Autodesk Inventor part; units mm, degrees
ref_plane "YZ Plane" through (0, 0, 0) normal (1, 0, 0) x (0, 1, 0)
ref_plane "XZ Plane" through (0, 0, 0) normal (0, 1, 0) x (-1, 0, 0)
ref_plane "XY Plane" through (0, 0, 0) normal (0, 0, 1) x (1, 0, 0)
sketch "Sketch1" plane through (0, 0, 0) normal (0, 0, 1) x (1, 0, 0)
  line L0 (-40.9154, -1.8235) -> (49.0846, -1.8235)
  line L1 (49.0846, -1.8235) -> (49.0846, -3.8235)
  line L2 (49.0846, -3.8235) -> (-40.9154, -3.8235)
  line L3 (-40.9154, -3.8235) -> (-40.9154, -1.8235)
  line L4 (-40.9154, -1.8235) -> (-33.9154, -1.8235)
  line L5 (-33.9154, -1.8235) -> (-33.9154, 15.1765)
  line L6 (-33.9154, 15.1765) -> (-40.9154, 15.1765)
  line L7 (-40.9154, 15.1765) -> (-40.9154, -1.8235)
  line L8 (49.0846, -1.8235) -> (43.0846, -1.8235)
  line L9 (43.0846, -1.8235) -> (43.0846, 15.1765)
  line L10 (43.0846, 15.1765) -> (49.0846, 15.1765)
  line L11 (49.0846, 15.1765) -> (49.0846, -1.8235)
  circle A0 centre (-36.9154, 6.1765) radius 1.5
  circle A1 centre (46.0846, 11.1765) radius 1.5
  circle A2 centre (46.0846, 1.1765) radius 1.5
  point P0 (0, 0)
  point P1 (43.0846, -1.8235)
  point P2 (43.0846, -1.8235)
  dimension "d0" = 2
  dimension "d1" = 90
  dimension "d2" = 10
  dimension "d3" = 5
  dimension "d4" = 15
  dimension "d5" = 83
  dimension "d6" = 83
  dimension "d7" = 4
  dimension "d8" = 3
  dimension "d9" = 3
  dimension "d10" = 3
  dimension "d11" = 19
  dimension "d12" = 3
  dimension "d13" = 3
  dimension "d14" = 3
extrude "Extrusion1" add sketch "Sketch1" against normal blind 10 contours L7 L6 L5 L0 | L0 L1 L2 L3 | L9 L10 L11 L0 | A0 | A1 | A2
fillet "Fillet1" radius 2 2 edges at (-37.4154, 15.1765, 0) (46.0846, 15.1765, 0)
sketch "Sketch2" plane through (0, 0, 0) normal (0, 0, 1) x (1, 0, 0)
  line L0 (-40.9154, -3.8235) -> (49.0846, -3.8235)
  line L1 (-40.9154, 13.1765) -> (-40.9154, -3.8235)
  line L2 (49.0846, -3.8235) -> (49.0846, 13.1765)
  point P0 (0, 0)
  point P1 (-36.9154, 6.1765)
  point P2 (46.0846, 1.1765)
  point P3 (46.0846, 11.1765)
  dimension "d18" = 10
  dimension "d19" = 5
  dimension "d20" = 15
  dimension "d21" = 4
  dimension "d22" = 83
  dimension "d23" = 83
  dimension "d24" = 3
hole "Hole1" at (-36.9154, 6.1765, 0) at (46.0846, 1.1765, 0) at (46.0846, 11.1765, 0) direction (0, 0, -1) diameter 3 depth 10 tip angle 118
chamfer "Chamfer1" distance 2 angle 45 2 edges at (-33.9154, -1.8235, -5) (43.0846, -1.8235, -5)
sketch "Sketch3" plane through (-31.9154, -1.8235, 0) normal (0, 1, 0) x (1, 0, 0)
  line L0 (73, 0) -> (0, 0)
  line L1 (73, 10) -> (73, 0)
  point P0 (31.9154, 0)
  point P1 (23, 3.2)
  point P2 (63, 3.2)
  point P3 (68.374, 17.0038)
  dimension "d35" = 3.2
  dimension "d36" = 3.2
  dimension "d37" = 10
  dimension "d38" = 50
hole "Hole2" at (-8.9154, -1.8235, -3.2) at (31.0846, -1.8235, -3.2) at (36.4586, -1.8235, -17.0038) direction (0, -1, 0) diameter 3 depth 10 tip angle 118
sketch "Sketch4" plane through (-31.9154, -1.8235, 0) normal (0, 1, 0) x (1, 0, 0)
  line L0 (0, 10) -> (73, 10)
  line L1 (31, 10) -> (51, 10)
  line L2 (51, 10) -> (51, 3)
  line L3 (51, 3) -> (31, 3)
  line L4 (31, 3) -> (31, 10)
  circle A0 centre (23, 3.2) radius 1.5
  circle A1 centre (63, 3.2) radius 1.5
  line L5 (73, 0) -> (0, 0)
  point P0 (31.9154, 0)
  dimension "d46" = 8
  dimension "d47" = 12
  dimension "d48" = 3
extrude "Extrusion2" cut sketch "Sketch4" against normal blind 2 contours L0 L2 L3 L4
fillet "Fillet2" radius 2 2 edges at (-0.9154, -2.8235, -3) (19.0846, -2.8235, -3)
properties part number "atx-adapter_mount"
For this review, take the finished solid that the model builds, in its own axes (mm). A direction names the side the tool comes from. Give positions to 0.01 mm unless a question says otherwise; leave off trailing zeros. Loops run counter-clockwise (first coordinate to the right, second up) from the corner with the lowest first, then second, coordinate; pieces in that order, holes last. Notation, with made-up numbers: M -15.75,52 L 9.25,52 A21 cw 9.25,81 Z; hole C 36.25,45 d4. An arc over 180 degrees is marked long. Put each result on its own line as item: value. Start each with the question number.
(1) For pin 1 (5 mm diameter, centred on x = 19.5, z = -3.5, fed in from +Y); pin 2 (2.5 mm diameter, centred on x = 46.08, y = 1.18, fed in from +Z); pin 3 (1 mm diameter, centred on x = 11.5, y = -3, fed in from -Z), all flat-tipped, find the tip position at first contact; note any pin that passes through.
(2) Machinability: for faces 1 (the cylindrical face through (-37.464, 14.575, -0.57)), 2 (the flat face through (19.085, -3, -8)), 3 (the flat face through (4.1, -1.824, -2.7)), which of the approach directions +Z, -Z, +X, -X, +Y, -Y give a long, thin tool a straight path to every point of the face, cutting with its end or side? Answer none if there is none.
(3) The part is to be moulded in two halves that separate along Y. For faces 4 (the cylindrical face through (-0.314, -2.838, -3.57)), 5 (the cylindrical face through (46.997, 2.367, -5.07)), 6 (the flat face through (46, 15.176, -6)), say which applies: +Y half, -Y half, draft (parallel to the pull), parting line (faces both ways), or undercut.
(4) Add section B-B, the plane z = -6.5. Write out the cut boundary in (x, y), then the cut area to 3 significant figures.
(5) Add section D-D, the plane x = 11. Write out the cut boundary in (y, z).
(6) Wall thickness on L1, parallel to X at y = 1.25, z = -8.25; L2, parallel to X at y = -2, z = -3.25; L3, parallel to X at y = 13, z = -6.5: over which ranges is each line inside the solid? List them lowest first.
(7) Add section A-A, the plane y = 10.5. Write out the cut boundary in (x, z), then the cut area to 3 significant figures.
(8) Add section C-C, the plane y = 1.25. Write out the cut boundary in (x, z), then the cut area to 3 significant figures.
Result:
1. pin 1: stops at y = -1.82
1. pin 2: passes through
1. pin 3: stops at z = -3
2. face 1: +Z, +X, -X, +Y
2. face 2: -Z, +Y, -Y
2. face 3: +Z, -Z, +Y
3. face 4: draft
3. face 5: undercut
3. face 6: +Y half
4. outline: M -40.92,-3.82 L -0.92,-3.82 L -0.92,-1.82 L -31.92,-1.82 L -33.92,0.18 L -33.92,15.18 L -40.92,15.18 Z; M 19.08,-3.82 L 49.08,-3.82 L 49.08,15.18 L 43.08,15.18 L 43.08,0.18 L 41.08,-1.82 L 19.08,-1.82 Z; hole C -36.92,6.18 d3; hole C 46.08,1.18 d3; hole C 46.08,11.18 d3
4. area: 344 mm^2
5. outline: M -3.82,-3 L -1.82,-3 L -1.82,0 L -3.82,0 Z
6. L1: x = -40.92 to -33.92, 43.08 to 44.59, 47.58 to 49.08
6. L2: x = -40.92 to -10.41, -7.42 to 0.12, 18.05 to 29.59, 32.58 to 49.08
6. L3: x = -40.92 to -33.92, 43.08 to 49.08
7. outline: M -40.92,-10 L -33.92,-10 L -33.92,0 L -40.92,0 Z; M 43.08,-10 L 44.75,-10 L 44.75,0 L 43.08,0 Z; M 47.42,-10 L 49.08,-10 L 49.08,0 L 47.42,0 Z
7. area: 103 mm^2
8. outline: M -40.92,-10 L -33.92,-10 L -33.92,0 L -40.92,0 Z; M 43.08,-10 L 44.59,-10 L 44.59,0 L 43.08,0 Z; M 47.58,-10 L 49.08,-10 L 49.08,0 L 47.58,0 Z
8. area: 100 mm^2
